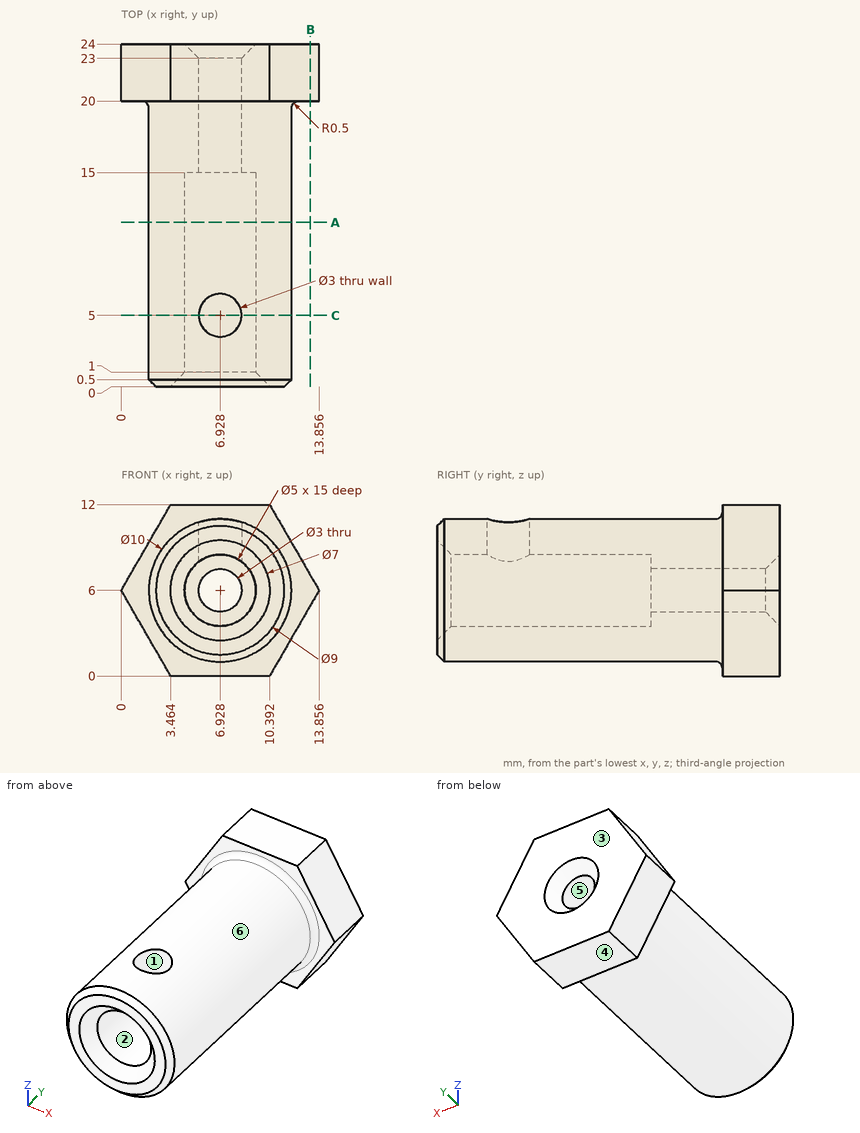
Answer from the drawing. Dimensions are ordinates in mm from the lowest x, y and z of the part. A direction names the side the tool comes from. Coordinates: 2 decimals unless noted, no trailing zeros. Order: outer loops, then holes, each group sorted by start corner. A loop starts at its lowest first (then second) coordinate and runs counter-clockwise, first axis right, second up. Notation, with made-up numbers: (6, -32) - (52, -32) arc R22 cw to (52, -6) - close; hole circle Ø3 at (7, 69.25). An arc over 180 degrees is marked (long way). Put each result on its own line as item: value. Start each with the question number.
1) Flat-ended cylindrical pins translate along their axes: pin 1 (8 mm diameter, centred on x = 8, y = 9, fed in from -Z); pin 2 (3.5 mm diameter, centred on x = 6.93, z = 6, fed in from -Y); pin 3 (5 mm diameter, centred on x = 4, y = 15, fed in from +Z). Find the tip coordinate at first contact, or state that the pin passes through.
2) For the marked faces 1, 2 and 3, determine the directions among +Z, -Z, +X, -X, +Y, -Y from which every point of the face is accessible in a straight line to the end or side of a thin tool.
3) For a pull along Z with two mould halves and no side action, classify the marked faces 4, 5 and 6 as released by +Z, released by -Z, zero draft, split by the parting line, or undercut.
4) Find section A-A (y = 11.5). Give the vertices of the cut face in (x, z).
5) Find the intervals of material crossed by line 1 (X direction, y = 10.5, z = 6); line 2 (X direction, y = 17.5, z = 6); line 3 (Z direction, x = 5.25, y = 5.25) (1 decimal), in increasing order. Write a range as from..to.
6) Find section B-B (x = 13.25). Give the vertices of the cut face in (y, z).
7) Find section C-C (y = 5). Give the vertices of the cut face in (x, z).
Results list:
1. pin 1: stops at z = 1
1. pin 2: stops at y = 15
1. pin 3: stops at z = 10.98
2. face 1: +Z
2. face 2: -Y
2. face 3: +Z, -Z, +X, -X, +Y
3. face 4: released by -Z
3. face 5: undercut
3. face 6: split by the parting line
4. outline: circle Ø10 at (6.93, 6); hole circle Ø5 at (6.93, 6)
5. line 1: x = 1.93..4.43, 9.43..11.93
5. line 2: x = 1.93..5.43, 8.43..11.93
5. line 3: z = 1.3..4.1, 7.9..10.7
6. outline: (20, 4.95) - (24, 4.95) - (24, 7.05) - (20, 7.05) - close
7. outline: (5.43, 8) - (5.43, 10.77) arc R5 ccw (long way) to (8.43, 10.77) - (8.43, 8) arc R2.5 cw (long way) to start
